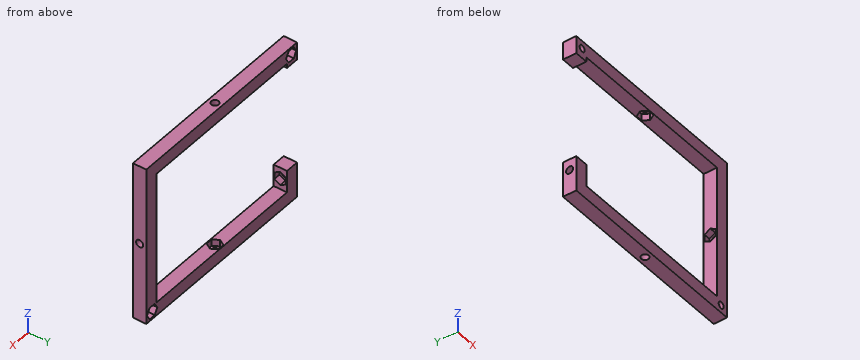
```python
from build123d import *

# Parameters (mm, degrees)
CROQUIS1_W              = 90
CROQUIS1_H              = 72
SALIENTE_EXTRUIR1_DEPTH = 6
CROQUIS2_R              = 1.5
CROQUIS2_W              = 78
CROQUIS2_H              = 60
CORTAR_EXTRUIR1_DEPTH   = 58.939623747
CORTAR_EXTRUIR2_DEPTH   = 3
CROQUIS4_R              = 1.625
CORTAR_EXTRUIR3_DEPTH   = 86.117565755
CORTAR_EXTRUIR4_REACH   = 99.118
CROQUIS5_R              = 1.625
CORTAR_EXTRUIR5_START   = -6
CROQUIS6_OUTSIDE_W      = 115.082
CROQUIS6_OUTSIDE_H      = 31.082
CROQUIS6_OUTSIDE_W_2    = 90
CROQUIS6_OUTSIDE_H_2    = 6
CORTAR_EXTRUIR5_DEPTH   = 3
CORTAR_EXTRUIR6_START   = -6
CORTAR_EXTRUIR6_DEPTH   = 3
CORTAR_EXTRUIR8_START   = -66
CROQUIS6_2_OUTSIDE_W    = 115.082
CROQUIS6_2_OUTSIDE_H    = 31.082
CROQUIS6_2_OUTSIDE_W_2  = 90
CROQUIS6_2_OUTSIDE_H_2  = 6
CORTAR_EXTRUIR8_DEPTH   = 3
CORTAR_EXTRUIR9_DEPTH   = 3
CORTAR_EXTRUIR10_REACH  = 93.586
CROQUIS10_R             = 1.625
CORTAR_EXTRUIR12_REACH  = 59.94
CROQUIS11_W             = 6
CROQUIS11_H             = 48


with BuildPart() as part:
    # Croquis1 → Saliente-Extruir1 (new body)
    with BuildSketch(Plane(origin=(0, 0, 0), x_dir=(1, 0, 0), z_dir=(0, 1, 0))):
        Rectangle(CROQUIS1_W, CROQUIS1_H)
    extrude(amount=SALIENTE_EXTRUIR1_DEPTH)

    # Croquis2 → Cortar-Extruir1 (cut, through all)
    with BuildSketch(Plane(origin=(0, 6, 0), x_dir=(1, 0, 0), z_dir=(0, 1, 0))):
        with Locations(Location((-41.5, -32.5, 0), (0, 0, 270))):
            Circle(CROQUIS2_R)
        with Locations(Location((41.5, 32.5, 0), (0, 0, 270))):
            Circle(CROQUIS2_R)
        Rectangle(CROQUIS2_W, CROQUIS2_H)
    extrude(amount=-CORTAR_EXTRUIR1_DEPTH, mode=Mode.SUBTRACT)

    # Croquis3 → Cortar-Extruir2 (cut)
    with BuildSketch(Plane(origin=(0, 6, 0), x_dir=(1, 0, 0), z_dir=(0, 1, 0))):
        Polygon((-39.970021787, -29.85), (-43.029978213, -29.85), (-44.559956427, -32.5), (-43.029978213, -35.15), (-39.970021787, -35.15), (-38.440043573, -32.5), align=None)
        Polygon((43.029978213, 35.15), (39.970021787, 35.15), (38.440043573, 32.5), (39.970021787, 29.85), (43.029978213, 29.85), (44.559956427, 32.5), align=None)
    extrude(amount=-CORTAR_EXTRUIR2_DEPTH, mode=Mode.SUBTRACT)

    # Croquis4 → Cortar-Extruir3 (cut, through all)
    with BuildSketch(Plane.XY.offset(36)):
        with Locations((0, 3)):
            Circle(CROQUIS4_R)
    extrude(amount=-CORTAR_EXTRUIR3_DEPTH, mode=Mode.SUBTRACT)

    # Croquis5 → Cortar-Extruir4 (cut, up to next)
    with BuildSketch(Plane(origin=(45, 0, 0), x_dir=(0, 0, -1), z_dir=(1, 0, 0)), mode=Mode.PRIVATE) as cortar_extruir4_sk1:
        with Locations((0, 3)):
            Circle(CROQUIS5_R)
    cortar_extruir4_tool1 = extrude(cortar_extruir4_sk1.sketch, amount=-CORTAR_EXTRUIR4_REACH, mode=Mode.PRIVATE) & part.part
    add(cortar_extruir4_tool1.solids().sort_by_distance((45, 3, 0))[0], mode=Mode.SUBTRACT)

    # Croquis6 outside → Cortar-Extruir5 (cut)
    # profile 1 of 2: a face of its own
    with BuildSketch(Plane.XY.offset(36).offset(CORTAR_EXTRUIR5_START)):
        with Locations((0, 3)):
            Rectangle(CROQUIS6_OUTSIDE_W, CROQUIS6_OUTSIDE_H)
        with Locations((0, 3)):
            Rectangle(CROQUIS6_OUTSIDE_W_2, CROQUIS6_OUTSIDE_H_2, mode=Mode.SUBTRACT)
    # profile 2 of 2: a face of its own
    with BuildSketch(Plane.XY.offset(36).offset(CORTAR_EXTRUIR5_START)):
        Polygon((1.529978213, 5.65), (-1.529978213, 5.65), (-3.059956427, 3), (-1.529978213, 0.35), (1.529978213, 0.35), (3.059956427, 3), align=None)
    extrude(amount=CORTAR_EXTRUIR5_DEPTH, mode=Mode.SUBTRACT)

    # Croquis8 → Cortar-Extruir6 (cut)
    with BuildSketch(Plane.ZY.offset(45).offset(CORTAR_EXTRUIR6_START)):
        Polygon((-23.470021787, 5.65), (-26.529978213, 5.65), (-28.059956427, 3), (-26.529978213, 0.35), (-23.470021787, 0.35), (-21.940043573, 3), align=None)
    extrude(amount=CORTAR_EXTRUIR6_DEPTH, mode=Mode.SUBTRACT)

    # Croquis6<2> outside → Cortar-Extruir8 (cut)
    # profile 1 of 2: a face of its own
    with BuildSketch(Plane.XY.offset(36).offset(CORTAR_EXTRUIR8_START)):
        with Locations((0, 3)):
            Rectangle(CROQUIS6_2_OUTSIDE_W, CROQUIS6_2_OUTSIDE_H)
        with Locations((0, 3)):
            Rectangle(CROQUIS6_2_OUTSIDE_W_2, CROQUIS6_2_OUTSIDE_H_2, mode=Mode.SUBTRACT)
    # profile 2 of 2: a face of its own
    with BuildSketch(Plane.XY.offset(36).offset(CORTAR_EXTRUIR8_START)):
        Polygon((1.529978213, 5.65), (-1.529978213, 5.65), (-3.059956427, 3), (-1.529978213, 0.35), (1.529978213, 0.35), (3.059956427, 3), align=None)
    extrude(amount=-CORTAR_EXTRUIR8_DEPTH, mode=Mode.SUBTRACT)

    # Croquis9 → Cortar-Extruir9 (cut)
    with BuildSketch(Plane.ZY.offset(-39)):
        Polygon((1.529978213, 5.65), (-1.529978213, 5.65), (-3.059956427, 3), (-1.529978213, 0.35), (1.529978213, 0.35), (3.059956427, 3), align=None)
    extrude(amount=-CORTAR_EXTRUIR9_DEPTH, mode=Mode.SUBTRACT)

    # Croquis10 → Cortar-Extruir10 (cut, up to next)
    with BuildSketch(Plane(origin=(-39, 0, 0), x_dir=(0, 0, -1), z_dir=(1, 0, 0)), mode=Mode.PRIVATE) as cortar_extruir10_sk1:
        with Locations((25, 3)):
            Circle(CROQUIS10_R)
    cortar_extruir10_tool1 = extrude(cortar_extruir10_sk1.sketch, amount=-CORTAR_EXTRUIR10_REACH, mode=Mode.PRIVATE) & part.part
    add(cortar_extruir10_tool1.solids().sort_by_distance((-39, 3, -25))[0], mode=Mode.SUBTRACT)

    # Croquis11 → Cortar-Extruir12 (cut, up to next)
    with BuildSketch(Plane(origin=(0, 6, 0), x_dir=(1, 0, 0), z_dir=(0, 1, 0)), mode=Mode.PRIVATE) as cortar_extruir12_sk1:
        with Locations((-42, -4)):
            Rectangle(CROQUIS11_W, CROQUIS11_H)
    cortar_extruir12_tool1 = extrude(cortar_extruir12_sk1.sketch, amount=-CORTAR_EXTRUIR12_REACH, mode=Mode.PRIVATE) & part.part
    add(cortar_extruir12_tool1.solids().sort_by_distance((-42, 6, 4))[0], mode=Mode.SUBTRACT)


solid = part.part
```
Work out the finished part from the listing and answer in its coordinate system (mm). Round coordinates to 2 decimals unless told otherwise and drop trailing zeros. Write each loop counter-clockwise with the first axis right and the second up, starting at its lowest first coordinate (ties: lowest second). Pieces come first, ordered by that corner, then holes.
1) A cutting plane is placed at C-C on z = 0. Determine the outline of the cut face in (x, y) (3 decimals).
2) A cutting plane is placed at B-B on x = -22. Determine the outline of the cut face in (y, z).
3) Flat-ended cylindrical pins translate along their axes: P1, Ø2.5, axis at x = 0, z = -32, coming from the -Y side; P2, Ø10, axis at x = -15.5, z = 22, coming from the -Y side; P3, Ø5, axis at x = 41.5, z = -32.5, coming from the +Y side; P4, Ø2, axis at y = 1, z = 0.5, coming from the -X side. Find the tip coordinate at first contact, or state that the pin passes through.
4) A cutting plane is placed at A-A on z = -25. Determine the outline of the cut face in (x, y) (3 decimals), and give its area (4 significant figures).
5) Consider probe 1 along Z at (x, y) = (24, 1.85); probe 2 along Y at (x, z) = (0, -35.4) (3 decimals); probe 3 along X at (y, z) = (1.5, 32). Determine where each line is inside the solid, lowest interval first.
Entries:
1. outline: (39, 0) - (45, 0) - (45, 1.375) - (42, 1.375) - (42, 0.35) - (39, 0.35) - close; (39, 5.65) - (42, 5.65) - (42, 4.625) - (45, 4.625) - (45, 6) - (39, 6) - close
2. outline: (0, -36) - (6, -36) - (6, -30) - (0, -30) - close; (0, 30) - (6, 30) - (6, 36) - (0, 36) - close
3. P1: stops at y = 0
3. P2: passes through
3. P3: stops at y = 3
3. P4: stops at x = 39
4. outline: (-45, 0) - (-39, 0) - (-39, 0.35) - (-42, 0.35) - (-42, 1.375) - (-45, 1.375) - close; (-45, 4.625) - (-42, 4.625) - (-42, 5.65) - (-39, 5.65) - (-39, 6) - (-45, 6) - close; (39, 0) - (45, 0) - (45, 6) - (39, 6) - close
4. area: 46.35 mm2
5. probe 1: z = -36 to -30, 30 to 36
5. probe 2: y = 0 to 1.375, 4.625 to 6
5. probe 3: x = -45 to -42.91, -40.09 to -2.19, 2.19 to 45
